Geometry: see drawing. Coordinates: mm, zero at the bounding-box minimum. Give positions to 0.01 mm unless a question says otherwise; leave off trailing zeros. Write each loop counter-clockwise with the first axis right and the second up, starting at its lowest first coordinate (ties: lowest second). Pieces come first, ordered by that corner, then holes. Notation, with made-up numbers: (39.5, -29) -> (64.5, -29) arc R34 ccw to (64.5, 10) -> close; hole circle Ø6 at (56.25, -9.5). An arc over 180 degrees is marked (long way). Use CSV: the item, a comma, the result in double quotes. Start each with the question number.
1) Contact query for flat-ended pins moving along their axis: P1, Ø0.5, axis at y = 0.5, z = 14, coming from the -X side; P2, Ø0.8, axis at y = 1, z = 16.5, coming from the -X side (1 decimal); P3, Ø0.8, axis at y = 1, z = 16.5, coming from the +X side (1 decimal). Output: stop coordinate, or through.
2) Material intervals for line 1 (Z direction, x = 109.22, y = 0.65); line 2 (X direction, y = 0.6, z = 11.5) (1 decimal); line 3 (X direction, y = 1.05, z = 18.25) (1 decimal), sorted ascending. Write a range as [from, to].
3) Section B-B (x = 109.22). Output: boundary loops of the cut face in (y, z).
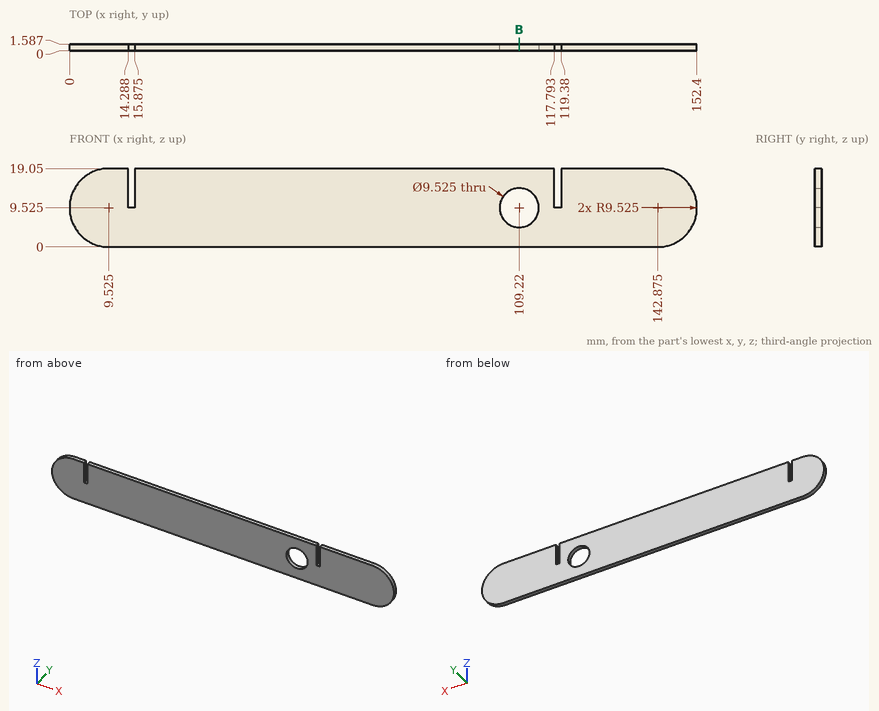
Answers follow:
1,P1,"stops at x = 0.99"
1,P2,"stops at x = 2.6"
1,P3,"stops at x = 149.8"
2,line 1,"z = [0, 4.76], [14.29, 19.05]"
2,line 2,"x = [0.2, 14.3], [15.9, 104.9], [113.6, 117.8], [119.4, 152.2]"
2,line 3,"x = [5.7, 14.3], [15.9, 117.8], [119.4, 146.7]"
3,outline,"(0, 0) -> (1.59, 0) -> (1.59, 4.76) -> (0, 4.76) -> close; (0, 14.29) -> (1.59, 14.29) -> (1.59, 19.05) -> (0, 19.05) -> close"
